from build123d import *

# Parameters (mm, degrees)
F0_W     = 116.7918927968
F0_H     = 80.2520625293
F1_DEPTH = 63.5
F2_R     = 12.7
F3_T     = 7.62


# Not quite as in the source:
# - a shell that OpenCascade refuses in one call is made with other operations: the cavity is built on its own and cut out


with BuildPart() as f1:
    # F0 (on Front) → F1 (new body, symmetric)
    with BuildSketch(Plane.XZ):
        with Locations((1.3399217278, 3.6678072065)):
            Rectangle(F0_W, F0_H)
    extrude(amount=F1_DEPTH, both=True)

    # F2
    f2_edges = [f1.edges().sort_by_distance(p)[0] for p in [
        (-57.056025, 0, 43.793838),
        (1.339922, 63.5, 43.793838),
        (59.735868, 0, 43.793838),
        (-57.056025, -63.5, 3.667807),
        (-57.056025, 63.5, 3.667807),
        (59.735868, -63.5, 3.667807),
        (59.735868, 63.5, 3.667807),
        (1.339922, 63.5, -36.458224),
        (1.339922, -63.5, -36.458224),
        (-57.056025, 0, -36.458224),
        (1.339922, -63.5, 43.793838),
    ]]
    fillet(f2_edges, radius=F2_R)

    # F3: shell of thickness 7.62, made by hand


with BuildPart() as f3_core1:
    # F3_t2: copy of F1
    add(f1.part)

    # the walls: a layer under each face that stays
    f3_faces = [f3_core1.faces().sort_by_distance(p)[0] for p in [
        (-53.3362807917, 0, 40.0740945922),
        (1.3399217278, 59.7802561211, 40.0740945922),
        (1.3399217278, -59.7802561211, 40.0740945922),
        (-50.7060246706, 59.7802561211, 37.4438384712),
        (-50.7060246706, -59.7802561211, 37.4438384712),
        (-57.0560246706, 0, 3.6678072065),
        (56.0161242472, 57.15, 37.4438384712),
        (1.3399217278, 63.5, 3.6678072065),
        (53.3858681262, -59.7802561211, 37.4438384712),
        (1.3399217278, -63.5, 3.6678072065),
        (-53.3362807917, 59.7802561211, 3.6678072065),
        (-53.3362807917, -59.7802561211, 3.6678072065),
        (-53.3362807917, 0, -32.7384801792),
        (56.0161242472, 59.7802561211, -2.6821927935),
        (7.6899217278, 59.7802561211, -32.7384801792),
        (56.0161240867, -59.7802562816, -2.6821927935),
        (7.6899217278, -59.7802562816, -32.7384800187),
        (7.6899217278, 0, -36.4582240582),
        (-50.7060246706, 57.15, -32.7384801792),
        (-50.7060246706, -57.15, -32.7384801792),
    ]]
    thicken(f3_faces, amount=-F3_T, mode=Mode.SUBTRACT)


with BuildPart() as f1_1:
    add(f1.part)

    # what is left inside the walls is the cavity
    f3_cavity = [f3_core1.part.solids().sort_by_distance(p)[0] for p in [
        (7.689922, 16.933333, -28.762024),
    ]]
    add(f3_cavity, mode=Mode.SUBTRACT)


solid = f1_1.part
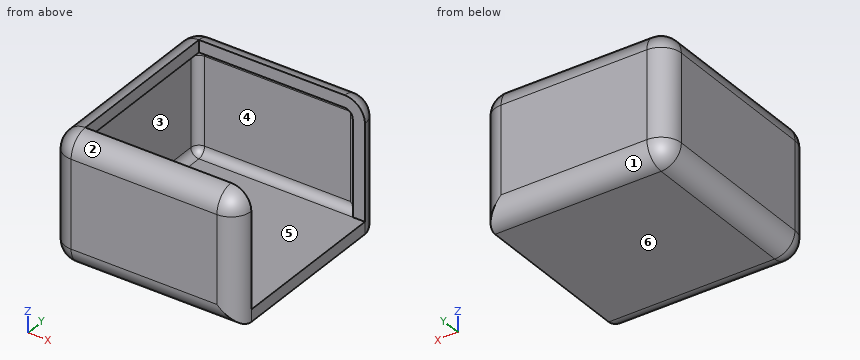
Geometry check sheet. Reference: the model listing, model coordinates, mm. Face numbers are marked on the shaded views. A direction names the side the tool comes from. Give positions to 0.01 mm unless a question says otherwise; leave off trailing zeros. Order: outer loops, then holes, each group sorted by start corner. A loop starts at its lowest first (then second) coordinate and runs counter-clockwise, first axis right, second up.
1. Scan lines: line 1 (Y direction, x = 12, z = -11); line 2 (X direction, y = 8, z = 3.5); line 3 (Z direction, x = 3, y = -41.5). Record each from-to range of solid material in increasing order.
Completed:
line 1: y = -63.5 to -55.88, 55.88 to 63.5
line 2: x = -57.06 to -49.44
line 3: z = -36.46 to -28.84
2. Sectioned sample at D-D (x = -47). Record the boundary of the cut face in (y, z).
Completed:
outline: (-63.22, -23.76) arc R12.42 ccw to (-50.8, -36.18) - (50.8, -36.18) arc R12.42 ccw to (63.22, -23.76) - (63.22, 31.09) arc R12.42 ccw to (50.8, 43.52) - (-50.8, 43.52) arc R12.42 ccw to (-63.22, 31.09) - close; hole (-55.14, -23.76) arc R4.34 ccw to (-50.8, -28.1) - (50.8, -28.1) arc R4.34 ccw to (55.14, -23.76) - (55.14, 31.09) arc R4.34 ccw to (50.8, 35.43) - (-50.8, 35.43) arc R4.34 ccw to (-55.14, 31.09) - close
3. Draft check along Y on the marked faces 1, 2 and 3. Enter one of: pulls with the +Y half, pulls with the -Y half, needs draft (parallel to the pull), parting line crosses it, or undercut.
Completed:
face 1: pulls with the +Y half
face 2: pulls with the -Y half
face 3: undercut
4. Sectioned sample at B-B (x = -27.5). Record the boundary of the cut face in (y, z), then the cut area to 3 significant figures.
Completed:
outline: (-63.5, -23.76) arc R12.7 ccw to (-50.8, -36.46) - (50.8, -36.46) arc R12.7 ccw to (63.5, -23.76) - (63.5, 31.09) arc R12.7 ccw to (50.8, 43.79) - (50.8, 36.17) arc R5.08 cw to (55.88, 31.09) - (55.88, -23.76) arc R5.08 cw to (50.8, -28.84) - (-50.8, -28.84) arc R5.08 cw to (-55.88, -23.76) - (-55.88, 31.09) arc R5.08 cw to (-50.8, 36.17) - (-50.8, 43.79) arc R12.7 ccw to (-63.5, 31.09) - close
area: 2,040 mm2
5. Sectioned sample at C-C (y = -8.5). Record the boundary of the cut face in (x, z).
Completed:
outline: (-57.06, -23.76) arc R12.7 ccw to (-44.36, -36.46) - (59.74, -36.46) - (59.74, -28.84) - (-44.36, -28.84) arc R5.08 cw to (-49.44, -23.76) - (-49.44, 31.09) arc R5.08 cw to (-44.36, 36.17) - (-44.36, 43.79) arc R12.7 ccw to (-57.06, 31.09) - close
6. Depth check by flat-ended pin: pin 1 (6 mm diameter, centred on y = 3.5, z = 38.5, fed in from +X); pin 2 (5 mm diameter, centred on x = 29, y = -8, fed in from +Z); pin 3 (1.5 mm diameter, centred on y = -23, z = 31, fed in from +X). Enter the tip coordinate at first touch or a pass-through.
Completed:
pin 1: stops at x = -44.36
pin 2: stops at z = -28.84
pin 3: stops at x = -49.39
7. Sectioned sample at A-A (z = 18). Record the boundary of the cut face in (x, y).
Completed:
outline: (-57.06, -50.8) arc R12.7 ccw to (-44.36, -63.5) - (47.04, -63.5) arc R12.7 ccw to (59.74, -50.8) - (52.12, -50.8) arc R5.08 cw to (47.04, -55.88) - (-44.36, -55.88) arc R5.08 cw to (-49.44, -50.8) - (-49.44, 50.8) arc R5.08 cw to (-44.36, 55.88) - (47.04, 55.88) arc R5.08 cw to (52.12, 50.8) - (59.74, 50.8) arc R12.7 ccw to (47.04, 63.5) - (-44.36, 63.5) arc R12.7 ccw to (-57.06, 50.8) - close
8. Access from +Z, -Z, +X, -X, +Y, -Y to the whole of each face (thin tool, end or side, straight path). Record for the marked faces 4, 5 and 6.
Completed:
face 4: none
face 5: +Z, +X
face 6: -Z, +X, -X, +Y, -Y
